Part model, mm, in its own coordinate system. Face numbers are marked on the shaded views. Give positions to 0.01 mm unless a question says otherwise; leave off trailing zeros. Order: outer loops, then holes, each group sorted by start corner. A loop starts at its lowest first (then second) coordinate and runs counter-clockwise, first axis right, second up. Notation, with made-up numbers: (65, 87.5) -> (89, 87.5) arc R9 cw to (89, 100.5) -> close; hole circle Ø6 at (77, 66.25). An arc over 180 degrees is marked (long way). Write item = value, one per line. Start each with the question number.
Item 1: Drill centre lines: line 1 along Y through (x, z) = (0, 2.5); line 2 along Z through (x, y) = (-11, 11); line 3 along X through (y, z) = (-4.5, 1.75). Where is each one in solid material? Low to high.
Item 2: Flat gauge pins, fed straight in: P1, Ø10, axis at x = 3.5, y = -9.5, coming from the -Z side; P2, Ø1.5, axis at x = 9.5, z = 8.5, coming from the +Y side; P3, Ø0.8, axis at x = -13, y = -13.5, coming from the -Z side; P4, Ø0.8, axis at y = -14, z = 1, coming from the -X side. Where does each tip first touch, or does it go through?
Item 3: Band-saw the part on C-C on y = 3. Write the cut outline in (x, z), plus the area to 3 significant figures.
Item 4: Band-saw the part on A-A on x = 0. Write the cut outline in (y, z), plus the area to 3 significant figures.
Item 5: Band-saw the part on B-B on z = 7. Write the cut outline in (x, y), plus the area to 3 significant figures.
Item 6: Pull direction X, two halves, no side cores. Call the marked faces 1, 2, 3 and 4: +X half, -X half, draft (parallel to the pull), parting line (faces both ways), or undercut.
Item 7: Band-saw the part on D-D on z = 4.5. Write the cut outline in (x, y).
```python
from build123d import *

# Parameters (mm, degrees)
F0_W          = 40
F0_H          = 40
F1_DEPTH      = 10
F3_DEPTH      = 0.5
F4_R          = 4.1
F5_DEPTH      = 10.001
F7_W          = 2.5
F7_H          = 2.75
F8_DEPTH      = 15
F11_REACH     = 43.3551019662
F12_R         = 1.5
F13_DEPTH     = 10.0010001
F14_T1_DEPTH  = 17.5
F14_T3_DEPTH  = 47.5
F14_T5_DEPTH  = 30
F14_T7_DEPTH  = 30
F14_T9_DEPTH  = 47.5
F14_S13_W     = 5
F14_S13_H     = 5
F14_T14_DEPTH = 5
F14_S19_W     = 5
F14_S19_H     = 5
F14_T20_DEPTH = 5
F14_S25_W     = 5
F14_S25_H     = 5
F14_T26_DEPTH = 5


# Not quite as in the source:
# - a fillet or chamfer that OpenCascade refuses, or shapes differently, is made with other operations: its cross-section is extruded or revolved along the edge and cut away or added


with BuildPart() as f1:
    # F0 (on Top) → F1 (new body)
    with BuildSketch(Plane.XY):
        Rectangle(F0_W, F0_H)
    extrude(amount=F1_DEPTH)

    # F2 (on face) → F3 (cut)
    with BuildSketch(Plane(origin=(0, 0, 0), x_dir=(1, 0, 0), z_dir=(0, 0, -1))):
        Polygon((11.3946354911, 9.8654455945), (-14.7593317032, -5.2345544055), (-14.7593317032, -20), (-5.3464073564, -20), (11.3946354911, -10.3345544055), align=None)
    extrude(amount=-F3_DEPTH, mode=Mode.SUBTRACT)

    # F4 (on face) → F5 (cut, through all)
    with BuildSketch(Plane(origin=(0, 0, 0), x_dir=(1, 0, 0), z_dir=(0, 0, -1))):
        with Locations((-10.6475949287, 6.1114258133)):
            Circle(F4_R)
    extrude(amount=-F5_DEPTH, mode=Mode.SUBTRACT)

    # F7 (on face) → F8 (cut)
    with BuildSketch(Plane(origin=(-20, 0, 0), x_dir=(0, -1, 0), z_dir=(-1, 0, 0))):
        with Locations((13.6307496577, 1.375)):
            Rectangle(F7_W, F7_H)
    extrude(amount=-F8_DEPTH, mode=Mode.SUBTRACT)

    f11_end = f1.faces().sort_by_distance((-14.7475949287, -6.1114258133, 5))[0]
    # F10 (on face) → F11 (cut, up to a face of the model that its end follows)
    with BuildSketch(Plane.XZ.offset(20)):
        with BuildLine():
            Line((-12.1130503118, 0), (-9.1130503118, 0))
            ThreePointArc((-9.1130503118, 0), (-10.6130503118, 1.5), (-12.1130503118, 0))
        make_face()
    f11_long = extrude(amount=-F11_REACH, mode=Mode.PRIVATE)
    add(split(f11_long, bisect_by=f11_end, keep=Keep.ALL, mode=Mode.PRIVATE).solids().sort_by_distance((-10.6130503118, -20, 0.6366197724))[0], mode=Mode.SUBTRACT)

    # F12 (on face) → F13 (cut, through all)
    with BuildSketch(Plane(origin=(0, 0, 0), x_dir=(1, 0, 0), z_dir=(0, 0, -1))):
        with Locations((0, 11.5903077688)):
            Circle(F12_R)
        with Locations((14.5839625479, -14.4456071497)):
            Circle(F12_R)
    extrude(amount=-F13_DEPTH, mode=Mode.SUBTRACT)

    # F14: fillet of radius 5 on 7 edges, made by hand

    # F14_s2 → F14_t1 (cut)
    with BuildSketch(Plane.XY.offset(-12.5)):
        with BuildLine():
            ThreePointArc((-15, -20), (-18.5355339059, -18.5355339059), (-20, -15))
            Line((-20, -15), (-20, -20))
            Line((-20, -20), (-15, -20))
        make_face()
        with BuildLine():
            ThreePointArc((-20, 15), (-18.5355339059, 18.5355339059), (-15, 20))
            Line((-15, 20), (-20, 20))
            Line((-20, 20), (-20, 15))
        make_face()
        with BuildLine():
            ThreePointArc((15, -20), (18.5355339059, -18.5355339059), (20, -15))
            Line((20, -15), (20, -20))
            Line((20, -20), (15, -20))
        make_face()
    extrude(amount=F14_T1_DEPTH, mode=Mode.SUBTRACT)

    # F14_s4 → F14_t3 (cut)
    with BuildSketch(Plane.XZ.offset(-32.5)):
        with BuildLine():
            ThreePointArc((20, 5), (18.5355339059, 8.5355339059), (15, 10))
            Line((15, 10), (20, 10))
            Line((20, 10), (20, 5))
        make_face()
    extrude(amount=F14_T3_DEPTH, mode=Mode.SUBTRACT)

    # F14_s6 → F14_t5 (cut)
    with BuildSketch(Plane.YZ.offset(-15)):
        with BuildLine():
            ThreePointArc((-20, 5), (-18.5355339059, 8.5355339059), (-15, 10))
            Line((-15, 10), (-20, 10))
            Line((-20, 10), (-20, 5))
        make_face()
    extrude(amount=F14_T5_DEPTH, mode=Mode.SUBTRACT)

    # F14_s8 → F14_t7 (cut)
    with BuildSketch(Plane.XZ.offset(-15)):
        with BuildLine():
            ThreePointArc((-15, 10), (-18.5355339059, 8.5355339059), (-20, 5))
            Line((-20, 5), (-20, 10))
            Line((-20, 10), (-15, 10))
        make_face()
    extrude(amount=F14_T7_DEPTH, mode=Mode.SUBTRACT)

    # F14_s10 → F14_t9 (cut)
    with BuildSketch(Plane.YZ.offset(-15)):
        with BuildLine():
            ThreePointArc((15, 10), (18.5355339059, 8.5355339059), (20, 5))
            Line((20, 5), (20, 10))
            Line((20, 10), (15, 10))
        make_face()
    extrude(amount=F14_T9_DEPTH, mode=Mode.SUBTRACT)


with BuildPart() as f14_tool12:
    # F14_s13 → F14_t14 (new body)
    with BuildSketch(Plane.XZ.offset(15)):
        with Locations((-17.5, 7.5)):
            Rectangle(F14_S13_W, F14_S13_H)
    extrude(amount=F14_T14_DEPTH)

    # F14_s15 → F14_t16 (revolve, cut)
    with BuildSketch(Plane(origin=(-15, -15, 5), x_dir=(0.7071067812, 0, -0.7071067812), z_dir=(-0.7071067812, 0, -0.7071067812))):
        with BuildLine():
            ThreePointArc((0, -5), (5, 0), (0, 5))
            Line((0, 5), (0, -5))
        make_face()
    revolve(axis=Axis((-15, -15, 5), (0, -1, 0)), mode=Mode.SUBTRACT)


with BuildPart() as f1_1:
    add(f1.part)

    # F14_t11: cut F14_tool12
    add(f14_tool12.part, mode=Mode.SUBTRACT)


with BuildPart() as f14_tool18:
    # F14_s19 → F14_t20 (new body)
    with BuildSketch(Plane.XZ.offset(-15)):
        with Locations((-17.5, 7.5)):
            Rectangle(F14_S19_W, F14_S19_H)
    extrude(amount=-F14_T20_DEPTH)

    # F14_s21 → F14_t22 (revolve, cut)
    with BuildSketch(Plane(origin=(-15, 15, 5), x_dir=(0.7071067812, 0, -0.7071067812), z_dir=(0.7071067812, 0, 0.7071067812))):
        with BuildLine():
            ThreePointArc((0, -5), (5, 0), (0, 5))
            Line((0, 5), (0, -5))
        make_face()
    revolve(axis=Axis((-15, 15, 5), (0, 1, 0)), mode=Mode.SUBTRACT)


with BuildPart() as f1_2:
    add(f1_1.part)

    # F14_t17: cut F14_tool18
    add(f14_tool18.part, mode=Mode.SUBTRACT)


with BuildPart() as f14_tool24:
    # F14_s25 → F14_t26 (new body)
    with BuildSketch(Plane.XZ.offset(15)):
        with Locations((17.5, 7.5)):
            Rectangle(F14_S25_W, F14_S25_H)
    extrude(amount=F14_T26_DEPTH)

    # F14_s27 → F14_t28 (revolve, cut)
    with BuildSketch(Plane(origin=(15, -15, 5), x_dir=(-0.7071067812, 0, -0.7071067812), z_dir=(-0.7071067812, 0, 0.7071067812))):
        with BuildLine():
            ThreePointArc((0, -5), (5, 0), (0, 5))
            Line((0, 5), (0, -5))
        make_face()
    revolve(axis=Axis((15, -15, 5), (0, -1, 0)), mode=Mode.SUBTRACT)


with BuildPart() as f1_3:
    add(f1_2.part)

    # F14_t23: cut F14_tool24
    add(f14_tool24.part, mode=Mode.SUBTRACT)


solid = f1_3.part
```
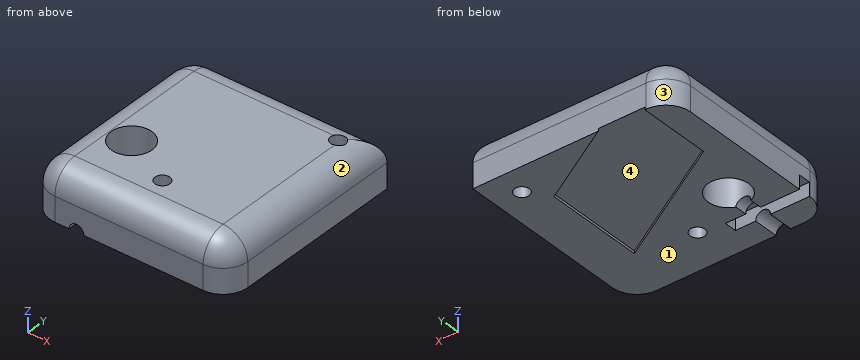
Values found:
q1.line_1 = -20 to -13.09, -10.09 to 20
q1.line_2 = 0.5 to 10
q1.line_3 = -20 to -14.42, -6.88 to 20
q2.P1 = 0
q2.P2 = 19.18
q2.P3 = 2.75
q2.P4 = -5
q3.outline = (-20, 0) -> (-10.89, 0) -> (-10.89, 0.5) -> (11.39, 0.5) -> (11.39, 0) -> (20, 0) -> (20, 5) arc R5 ccw to (15, 10) -> (-15, 10) arc R5 ccw to (-20, 5) -> close
q3.area = 378 mm^2
q4.outline = (-20, 0) -> (-13.09, 0) -> (-13.09, 10) -> (-15, 10) arc R5 ccw to (-20, 5) -> close; (-10.09, 0) -> (-3.29, 0) -> (-3.29, 0.5) -> (16.91, 0.5) -> (16.91, 0) -> (20, 0) -> (20, 5) arc R5 ccw to (15, 10) -> (-10.09, 10) -> close
q4.area = 349 mm^2
q5.outline = (-19.58, -15) arc R4.58 ccw to (-15, -19.58) -> (15, -19.58) arc R4.58 ccw to (19.58, -15) -> (19.58, 19.58) -> (-15, 19.58) arc R4.58 ccw to (-19.58, 15) -> close; hole circle Ø8.2 at (-10.65, -6.11); hole circle Ø3 at (0, -11.59); hole circle Ø3 at (14.58, 14.45)
q5.area = 1,450 mm^2
q6.face_1 = draft
q6.face_2 = +X half
q6.face_3 = -X half
q6.face_4 = undercut
q7.outline = (-20, -15) arc R5 ccw to (-15, -20) -> (15, -20) arc R5 ccw to (20, -15) -> (20, 20) -> (-15, 20) arc R5 ccw to (-20, 15) -> close; hole circle Ø8.2 at (-10.65, -6.11); hole circle Ø3 at (0, -11.59); hole circle Ø3 at (14.58, 14.45)
